from build123d import *

# Parameters (mm, degrees)
SKETCH_1_R           = 29
EXTRUDE_1_DEPTH      = 15
SKETCH_2_R           = 1.55
SKETCH_2_R_2         = 2.6
CUT_EXTRUDE_1_DEPTH  = 44.669211122
EXTRUDE_2_DEPTH      = 71
SKETCH_12_W          = 70
SKETCH_12_H          = 15
EXTRUDE_3_DEPTH      = 71
FILLET_5_R           = 10
SKETCH_22_W          = 71
SKETCH_22_H          = 103
CUT_EXTRUDE_11_DEPTH = 10
SKETCH_4_R           = 40
CUT_EXTRUDE_2_DEPTH  = 56
SKETCH_5_R           = 15.6
SKETCH_5_R_2         = 1.55
CUT_EXTRUDE_3_DEPTH  = 171.241005636
SKETCH_6_W           = 32.2
SKETCH_6_H           = 32.2
CUT_EXTRUDE_4_DEPTH  = 23.7
CUT_EXTRUDE_5_DEPTH  = 171.241005636
SKETCH_8_W           = 10
SKETCH_8_H           = 50
CUT_EXTRUDE_6_DEPTH  = 10
FILLET_1_R           = 10
FILLET_2_R           = 10
FILLET_3_R           = 10
SKETCH_17_R          = 22.5
CUT_EXTRUDE_7_DEPTH  = 7
SKETCH_18_R          = 24
CUT_EXTRUDE_8_DEPTH  = 0.5
EXTRUDE_START        = 10
SKETCH_19_R          = 12.5
SKETCH_19_R_2        = 1.55
SKETCH_19_R_3        = 2.6
EXTRUDE_5_DEPTH      = 10
SKETCH_20_R          = 3
CUT_EXTRUDE_9_DEPTH  = 3
SKETCH_23_R          = 1.5
CUT_EXTRUDE_12_DEPTH = 161.262160225
SKETCH_27_R          = 3
CUT_EXTRUDE_14_DEPTH = 3
SKETCH_28_W          = 10
SKETCH_28_H          = 6
EXTRUDE_6_DEPTH      = 5
FILLET_6_R           = 5
EXTRUDE_7_DEPTH      = 10
EXTRUDE_8_DEPTH      = 6


# Some blends are built 0.0001 mm under size
with BuildPart() as part:
    # Sketch 1 → Extrude 1 (new body)
    with BuildSketch(Plane.XY):
        Circle(SKETCH_1_R)
    extrude(amount=EXTRUDE_1_DEPTH)

    # Sketch 2 → Cut-Extrude 1 (cut, through all)
    with BuildSketch(Plane.XY.offset(15)):
        with Locations((-3.25, 5.629165125)):
            Circle(SKETCH_2_R)
        with Locations((3.25, 5.629165125)):
            Circle(SKETCH_2_R)
        with Locations((6.5, 0)):
            Circle(SKETCH_2_R)
        with Locations((3.25, -5.629165125)):
            Circle(SKETCH_2_R)
        Circle(SKETCH_2_R_2)
        with Locations((-3.25, -5.629165125)):
            Circle(SKETCH_2_R)
        with Locations((-6.5, 0)):
            Circle(SKETCH_2_R)
    extrude(amount=-CUT_EXTRUDE_1_DEPTH, mode=Mode.SUBTRACT)

    # Sketch 17 → Cut-Extrude 7 (cut)
    with BuildSketch(Plane.XY.offset(15)):
        Circle(SKETCH_17_R)
    extrude(amount=-CUT_EXTRUDE_7_DEPTH, mode=Mode.SUBTRACT)

    # Sketch 18 → Cut-Extrude 8 (cut)
    with BuildSketch(Plane.XY.offset(8)):
        Circle(SKETCH_18_R)
    extrude(amount=-CUT_EXTRUDE_8_DEPTH, mode=Mode.SUBTRACT)


with BuildPart() as body_2:
    # Sketch 3 → Extrude 2 (new body)
    with BuildSketch(Plane.XY):
        with BuildLine():
            ThreePointArc((-29, 0), (0, 29), (29, 0))
            Line((29, 0), (29, 95))
            Line((29, 95), (-9, 95))
            Line((-9, 95), (-9, 145))
            Line((-9, 145), (-29, 145))
            Line((-29, 145), (-29, 0))
        make_face()
    extrude(amount=EXTRUDE_2_DEPTH)

    # Sketch 12 → Extrude 3 (add)
    with BuildSketch(Plane.XY.offset(71)):
        with Locations((0, 34.5)):
            Rectangle(SKETCH_12_W, SKETCH_12_H)
    extrude(amount=-EXTRUDE_3_DEPTH)

    # Fillet 5
    # the kernel refuses this fillet: 10 mm, written as the material it takes off along each edge
    with BuildSketch(Plane(origin=(35, 42, 93.912878475), x_dir=(0, -1, 0), z_dir=(0, 0, -1))) as fillet_5_piece_1:
        with BuildLine():
            CenterArc((9.16515139, 10), FILLET_5_R, 203.578178478, 66.421821522)
            Line((0, 6), (-0.183303028, 5.92))
            ThreePointArc((-0.183303028, 5.92), (-0.2, 3), (-0.2, 0))
            Line((-0.2, 0), (0, -0.2))
            Line((0, -0.2), (9.16515139, -0.2))
            Line((9.16515139, -0.2), (9.16515139, 0))
        make_face()
    extrude(amount=116.82575695, mode=Mode.SUBTRACT)
    with BuildSketch(Plane(origin=(-35, 42, 93.912878475), x_dir=(0, -1, 0), z_dir=(0, 0, -1))) as fillet_5_piece_2:
        with BuildLine():
            CenterArc((9.16515139, -10), FILLET_5_R, 90, 66.421821522)
            Line((0, -6), (-0.183303028, -5.92))
            ThreePointArc((-0.183303028, -5.92), (-0.2, -3), (-0.2, 0))
            Line((-0.2, 0), (0, 0.2))
            Line((0, 0.2), (9.16515139, 0.2))
            Line((9.16515139, 0.2), (9.16515139, 0))
        make_face()
    extrude(amount=116.82575695, mode=Mode.SUBTRACT)

    # Sketch 22 → Cut-Extrude 11 (cut)
    with BuildSketch(Plane.ZY.offset(29)):
        with Locations((35.5, 93.5)):
            Rectangle(SKETCH_22_W, SKETCH_22_H)
    extrude(amount=-CUT_EXTRUDE_11_DEPTH, mode=Mode.SUBTRACT)

    # Sketch 4 → Cut-Extrude 2 (cut)
    with BuildSketch(Plane.XY.offset(71)):
        Circle(SKETCH_4_R)
    extrude(amount=-CUT_EXTRUDE_2_DEPTH, mode=Mode.SUBTRACT)

    # Sketch 5 → Cut-Extrude 3 (cut, through all)
    with BuildSketch(Plane.ZY.offset(19)):
        with Locations(Location((42.5, 70, 0), (0, 0, 270))):
            Circle(SKETCH_5_R)
        with Locations(Location((29.241747853, 83.258252147, 0), (0, 0, 270))):
            Circle(SKETCH_5_R_2)
        with Locations(Location((55.758252147, 83.258252147, 0), (0, 0, 270))):
            Circle(SKETCH_5_R_2)
        with Locations(Location((55.758252147, 56.741747853, 0), (0, 0, 270))):
            Circle(SKETCH_5_R_2)
        with Locations(Location((29.241747853, 56.741747853, 0), (0, 0, 270))):
            Circle(SKETCH_5_R_2)
    extrude(amount=-CUT_EXTRUDE_3_DEPTH, mode=Mode.SUBTRACT)

    # Sketch 6 → Cut-Extrude 4 (cut)
    with BuildSketch(Plane.ZY.offset(19)):
        with Locations((42.5, 70)):
            Rectangle(SKETCH_6_W, SKETCH_6_H)
    extrude(amount=-CUT_EXTRUDE_4_DEPTH, mode=Mode.SUBTRACT)

    # Sketch 7 → Cut-Extrude 5 (cut, through all)
    with BuildSketch(Plane.ZY.offset(19)):
        with BuildLine():
            Line((56.95, 137.497499937), (56.95, 133.497499937))
            ThreePointArc((56.95, 133.497499937), (58.5, 131.947499937), (60.05, 133.497499937))
            Line((60.05, 133.497499937), (60.05, 137.497499937))
            ThreePointArc((60.05, 137.497499937), (58.5, 139.047499937), (56.95, 137.497499937))
        make_face()
        with BuildLine():
            Line((54.1, 121.997499937), (54.1, 117.997499937))
            ThreePointArc((54.1, 117.997499937), (43, 106.897499937), (31.9, 117.997499937))
            Line((31.9, 117.997499937), (31.9, 121.997499937))
            ThreePointArc((31.9, 121.997499937), (43, 133.097499937), (54.1, 121.997499937))
        make_face()
        with BuildLine():
            Line((29.05, 137.497499937), (29.05, 133.497499937))
            ThreePointArc((29.05, 133.497499937), (27.5, 131.947499937), (25.95, 133.497499937))
            Line((25.95, 133.497499937), (25.95, 137.497499937))
            ThreePointArc((25.95, 137.497499937), (27.5, 139.047499937), (29.05, 137.497499937))
        make_face()
        with BuildLine():
            Line((56.95, 106.497499937), (56.95, 102.497499937))
            ThreePointArc((56.95, 102.497499937), (58.5, 100.947499937), (60.05, 102.497499937))
            Line((60.05, 102.497499937), (60.05, 106.497499937))
            ThreePointArc((60.05, 106.497499937), (58.5, 108.047499937), (56.95, 106.497499937))
        make_face()
        with BuildLine():
            Line((25.95, 106.497499937), (25.95, 102.497499937))
            ThreePointArc((25.95, 102.497499937), (27.5, 100.947499937), (29.05, 102.497499937))
            Line((29.05, 102.497499937), (29.05, 106.497499937))
            ThreePointArc((29.05, 106.497499937), (27.5, 108.047499937), (25.95, 106.497499937))
        make_face()
    extrude(amount=-CUT_EXTRUDE_5_DEPTH, mode=Mode.SUBTRACT)

    # Sketch 8 → Cut-Extrude 6 (cut)
    with BuildSketch(Plane(origin=(0, 0, 0), x_dir=(-1, 0, 0), z_dir=(0, 0, -1))):
        with Locations((14, 120)):
            Rectangle(SKETCH_8_W, SKETCH_8_H)
    extrude(amount=-CUT_EXTRUDE_6_DEPTH, mode=Mode.SUBTRACT)

    # Fillet 1
    fillet_1_edges = [body_2.edges().sort_by_distance(p)[0] for p in [
        (5, 95, 0),
    ]]
    fillet(fillet_1_edges, radius=FILLET_1_R)

    # Fillet 2
    fillet_2_edges = [body_2.edges().sort_by_distance(p)[0] for p in [
        (-14, 145, 10),
    ]]
    fillet(fillet_2_edges, radius=FILLET_2_R)

    # Fillet 3
    fillet_3_edges = [body_2.edges().sort_by_distance(p)[0] for p in [
        (-14, 145, 71),
    ]]
    fillet(fillet_3_edges, radius=FILLET_3_R)


    add(part.part)  # Extrude 5 merges part
    # Sketch 19 → Extrude 5 (add)
    with BuildSketch(Plane.XY.offset(7.5).offset(EXTRUDE_START)):
        Circle(SKETCH_19_R)
        with Locations((-3.25, -5.629165125)):
            Circle(SKETCH_19_R_2, mode=Mode.SUBTRACT)
        with Locations((3.25, -5.629165125)):
            Circle(SKETCH_19_R_2, mode=Mode.SUBTRACT)
        with Locations((6.5, 0)):
            Circle(SKETCH_19_R_2, mode=Mode.SUBTRACT)
        Circle(SKETCH_19_R_3, mode=Mode.SUBTRACT)
        with Locations((3.25, 5.629165125)):
            Circle(SKETCH_19_R_2, mode=Mode.SUBTRACT)
        with Locations((-3.25, 5.629165125)):
            Circle(SKETCH_19_R_2, mode=Mode.SUBTRACT)
        with Locations((-6.5, 0)):
            Circle(SKETCH_19_R_2, mode=Mode.SUBTRACT)
    extrude(amount=-EXTRUDE_5_DEPTH)

    # Sketch 20 → Cut-Extrude 9 (cut)
    with BuildSketch(Plane(origin=(0, 0, 0), x_dir=(-1, 0, 0), z_dir=(0, 0, -1))):
        with Locations((-3.25, 5.629165125)):
            Circle(SKETCH_20_R)
        with Locations((3.25, 5.629165125)):
            Circle(SKETCH_20_R)
        with Locations((-6.5, 0)):
            Circle(SKETCH_20_R)
        with Locations((-3.25, -5.629165125)):
            Circle(SKETCH_20_R)
        with Locations((3.25, -5.629165125)):
            Circle(SKETCH_20_R)
        with Locations((6.5, 0)):
            Circle(SKETCH_20_R)
    extrude(amount=-CUT_EXTRUDE_9_DEPTH, mode=Mode.SUBTRACT)

    # Sketch 23 → Cut-Extrude 12 (cut, through all)
    with BuildSketch(Plane(origin=(0, 0, 58.6), x_dir=(-1, 0, 0), z_dir=(0, 0, -1))):
        with Locations((-16, 80)):
            Circle(SKETCH_23_R)
        with Locations((9, 80)):
            Circle(SKETCH_23_R)
        with Locations((9, 55)):
            Circle(SKETCH_23_R)
        with Locations((-16, 55)):
            Circle(SKETCH_23_R)
    extrude(amount=-CUT_EXTRUDE_12_DEPTH, mode=Mode.SUBTRACT)

    # Sketch 27 → Cut-Extrude 14 (cut)
    with BuildSketch(Plane(origin=(29, 0, 0), x_dir=(0, 0, -1), z_dir=(1, 0, 0))):
        with Locations((-55.758252147, 83.258252147)):
            Circle(SKETCH_27_R)
        with Locations((-29.241747853, 83.258252147)):
            Circle(SKETCH_27_R)
        with Locations((-55.758252147, 56.741747853)):
            Circle(SKETCH_27_R)
        with Locations((-29.241747853, 56.741747853)):
            Circle(SKETCH_27_R)
    extrude(amount=-CUT_EXTRUDE_14_DEPTH, mode=Mode.SUBTRACT)

    # Sketch 28 → Extrude 6 (add)
    with BuildSketch(Plane(origin=(29, 0, 0), x_dir=(0, 0, -1), z_dir=(1, 0, 0))):
        with Locations((-63.1, 67)):
            Rectangle(SKETCH_28_W, SKETCH_28_H)
    extrude(amount=EXTRUDE_6_DEPTH)

    # Fillet 6
    fillet_6_edges = [body_2.edges().sort_by_distance(p)[0] for p in [
        (29, 64, 63.1),
    ]]
    fillet(fillet_6_edges, radius=FILLET_6_R - 0.0001)  # a hair under: the kernel refuses the full size

    # Sketch 29 → Extrude 7 (add)
    with BuildSketch(Plane(origin=(0, 0, 0), x_dir=(-1, 0, 0), z_dir=(0, 0, -1))):
        Polygon((19, 70), (29, 42), (19, 42), align=None)
    extrude(amount=-EXTRUDE_7_DEPTH)

    # Sketch 30 → Extrude 8 (add)
    with BuildSketch(Plane.XY.offset(71)):
        Polygon((-29, 42), (-19, 70), (-19, 42), align=None)
    extrude(amount=-EXTRUDE_8_DEPTH)


solid = body_2.part
Could you check a few things on this model? Use its own coordinates, in mm. A direction names the side the tool comes from. Give positions to 0.01 mm unless a question says otherwise; leave off trailing zeros. Write each loop counter-clockwise with the first axis right and the second up, starting at its lowest first coordinate (ties: lowest second). Pieces come first, ordered by that corner, then holes. Notation, with made-up numbers: (4, -21) -> (44, -21) arc R16 ccw to (44, -7) -> close; hole circle Ø6 at (59.5, 29.5). An arc over 180 degrees is marked (long way). Write each question's results on one line, items separated by ' | '. Start each with the question number.
Q1. Suppose I cut it at A-A, the plane z = 42.5. List the corners of the cut face in (x, y) for me.
Q2. I'm going to push flat-ended pins straight in: pin 1 Ø7 at (y, z) = (56.74, 29.24) entering from -X; pin 2 Ø3.5 at (x, y) = (3.25, 5.63) entering from -Z; pin 3 Ø3 at (x, y) = (3.25, -5.63) entering from -Z; pin 4 Ø11 at (x, y) = (-21.5, 49.5) entering from -Z. Where does each tip first touch, or does it pass through?
Q3. I need wall thicknesses on probe 1 along Y at (x, z) = (3.25, 1.5); probe 2 along Z at (x, y) = (-1, 57); probe 3 along Y at (x, z) = (-3.25, 11.75). Which ranges of each line are inside material? Lowest first, please.
Q4. Suppose I cut it at B-B, the plane z = 22.5. List the corners of the cut face in (x, y) for me, and give its area (3 significant figures).
Q5. We'd pull the mould along Z, two halves only. Please class faces 1 (the face through (11.923, 3.755, 12.57)), 2 (the face through (-14.1, 106.9, 43.2)), 3 (the face through (-14.07, 142.15, 67.99)): +Z half, -Z half, draft (parallel to the pull), parting line (faces both ways), or undercut.
Q6. Which directions (+Z, -Z, +X, -X, +Y, -Y) give clear straight access to the entire face, cutting with the end or side of a thin tool? Please do faces 4 (the face through (-22, 50, 65)), 5 (the face through (-14.07, 108.047, 27.534)), 6 (the face through (29, 13, 7)).
Outcome:
1) outline: (-35, 27) -> (-29.51, 27) arc R40 cw to (29.51, 27) -> (35, 27) -> (35, 32.83) arc R10 ccw to (29, 42) -> (29, 54.4) -> (4.7, 54.4) -> (4.7, 53.9) -> (-19, 53.9) -> (-19, 42) -> (-29, 42) arc R10 ccw to (-35, 32.83) -> close; (-19, 86.1) -> (4.7, 86.1) -> (4.7, 85.6) -> (29, 85.6) -> (29, 95) -> (-9, 95) -> (-9, 106.91) -> (-19, 106.91) -> close; (-19, 133.09) -> (-9, 133.09) -> (-9, 145) -> (-19, 145) -> close
2) pin 1: x = -19 | pin 2: z = 3 | pin 3: through | pin 4: z = 0
3) probe 1: -28.82 to -8.63, -2.63 to 2.63, 8.63 to 90.27 | probe 2: 0 to 26.4, 58.6 to 71 | probe 3: -28.82 to -22.26, -12.07 to -7.18, -4.08 to 4.08, 7.18 to 12.07, 22.26 to 95
4) outline: (-35, 27) -> (-29.51, 27) arc R40 cw to (29.51, 27) -> (35, 27) -> (35, 32.83) arc R10 ccw to (29, 42) -> (29, 95) -> (-9, 95) -> (-9, 145) -> (-19, 145) -> (-19, 42) -> (-29, 42) arc R10 ccw to (-35, 32.83) -> close | area: 3,530 mm2
5) face 1: draft | face 2: undercut | face 3: +Z half
6) face 4: -X, +Y | face 5: +X, -X | face 6: +Z, -Z, +X, -Y
